from build123d import *

# Parameters (mm, degrees)
F0_R      = 40
F1_DEPTH  = 10
F2_R      = 35
F3_DEPTH  = 3
F4_R      = 35
F5_DEPTH  = 3
F6_SIZE   = 1
F7_R      = 14.543107
F8_DEPTH  = 2
F9_R      = 11.723212
F10_DEPTH = 25


with BuildPart() as f1:
    # F0 (on Top) → F1 (new body)
    with BuildSketch(Plane.XY):
        Circle(F0_R)
    extrude(amount=F1_DEPTH)

    # F2 (on face) → F3 (cut)
    with BuildSketch(Plane.XY.offset(10)):
        Circle(F2_R)
    extrude(amount=-F3_DEPTH, mode=Mode.SUBTRACT)

    # F4 (on face) → F5 (cut)
    with BuildSketch(Plane(origin=(0, 0, 0), x_dir=(1, 0, 0), z_dir=(0, 0, -1))):
        Circle(F4_R)
    extrude(amount=-F5_DEPTH, mode=Mode.SUBTRACT)

    # F6
    f6_edges = [f1.edges().sort_by_distance(p)[0] for p in [
        (-35, 0, 10),
        (-40, 0, 10),
        (-40, 0, 0),
        (-35, 0, 0),
    ]]
    chamfer(f6_edges, length=F6_SIZE)

    # F7 (on face) → F8 (cut)
    with BuildSketch(Plane.XY.offset(7)):
        Circle(F7_R)
    extrude(amount=-F8_DEPTH, mode=Mode.SUBTRACT)

    # F9 (on face) → F10 (join)
    with BuildSketch(Plane.XY.offset(5)):
        with Locations((0, 1.236479)):
            Circle(F9_R)
    extrude(amount=F10_DEPTH)


solid = f1.part
The listing builds one solid part. Answer for the finished solid, in the listing's coordinates (mm). A direction names the side the tool comes from. Coordinates: 2 decimals unless noted, no trailing zeros. Write each loop counter-clockwise with the first axis right and the second up, starting at its lowest first coordinate (ties: lowest second). Pieces come first, ordered by that corner, then holes. Notation, with made-up numbers: (78.5, 52) -> (108.5, 52) arc R21 ccw to (108.5, 61) -> close; hole circle Ø6 at (18.5, -3). An arc over 180 degrees is marked (long way). One line per question, with ' | ' between items.
1. For a pull along Y with two mould halves and no side action, classify faces 4 (the cylindrical face through (-28, 21, 2)), 5 (the cylindrical face through (-8.67, -39.05, 4.94)), 6 (the flat face through (11.4, -34.5, 10)) as released by +Y, released by -Y, zero draft, split by the parting line, or undercut.
Verdict:
face 4: undercut | face 5: split by the parting line | face 6: zero draft
2. Given pin 1 Ø10 at (x, y) = (31, -28) entering from +Z; pin 2 Ø12 at (x, z) = (-0.5, 20) entering from -Y; pin 3 Ø12 at (y, z) = (-31, 7) entering from -X (3 decimals), each flat-ended and moving along its own axis, determine where each tip first touches the part or whether it passes through.
Verdict:
pin 1: stops at z = 10 | pin 2: stops at y = -10.49 | pin 3: stops at x = -31.225
3. Section B-B (y = 0) is taken. Determine the outline of the cut face in (x, z), and give its area (3 significant figures).
Verdict:
outline: (-40, 1) -> (-39, 0) -> (-36, 0) -> (-35, 1) -> (-35, 3) -> (35, 3) -> (35, 1) -> (36, 0) -> (39, 0) -> (40, 1) -> (40, 9) -> (39, 10) -> (36, 10) -> (35, 9) -> (35, 7) -> (14.54, 7) -> (14.54, 5) -> (11.66, 5) -> (11.66, 30) -> (-11.66, 30) -> (-11.66, 5) -> (-14.54, 5) -> (-14.54, 7) -> (-35, 7) -> (-35, 9) -> (-36, 10) -> (-39, 10) -> (-40, 9) -> close | area: 901 mm^2
4. Which of the six approach directions +Z, -Z, +X, -X, +Y, -Y give full straight-line access (tool end or side, diameter ignored) to faces 1 (the cylindrical face through (-3.153, -14.197, 6.014)), 2 (the flat face through (11.4, -34.5, 0)), 3 (the flat face through (0, 0, 3))?
Verdict:
face 1: +Z | face 2: -Z, +X, -X, +Y, -Y | face 3: -Z
5. Section C-C (z = 19.5) is taken. Determine the outline of the cut face in (x, y), and give its area (3 significant figures).
Verdict:
outline: circle Ø23.45 at (0, 1.24) | area: 432 mm^2
6. Straight lines are drawn through the part: line 1 (Y direction, x = 0, z = 8.5); line 2 (Y direction, x = 0, z = 1.65); line 3 (Z direction, x = -22, y = 6). For each, find the intervals that lie inside material, in ascending order.
Verdict:
line 1: y = -40 to -35, -10.49 to 12.96, 35 to 40 | line 2: y = -40 to -35, 35 to 40 | line 3: z = 3 to 7
7. Section A-A (x = 0) is taken. Determine the outline of the cut face in (y, z), and give its area (3 significant figures).
Verdict:
outline: (-40, 1) -> (-39, 0) -> (-36, 0) -> (-35, 1) -> (-35, 3) -> (35, 3) -> (35, 1) -> (36, 0) -> (39, 0) -> (40, 1) -> (40, 9) -> (39, 10) -> (36, 10) -> (35, 9) -> (35, 7) -> (14.54, 7) -> (14.54, 5) -> (12.96, 5) -> (12.96, 30) -> (-10.49, 30) -> (-10.49, 5) -> (-14.54, 5) -> (-14.54, 7) -> (-35, 7) -> (-35, 9) -> (-36, 10) -> (-39, 10) -> (-40, 9) -> close | area: 904 mm^2
